Verification items for the finished model (mm, model axes). A direction names the side the tool comes from. Give positions to 0.01 mm unless a question says otherwise; leave off trailing zeros. Loops run counter-clockwise (first coordinate to the right, second up) from the corner with the lowest first, then second, coordinate; pieces in that order, holes last. Notation, with made-up numbers: (3, -11) - (54, -11) arc R27 ccw to (54, 21) - close; hole circle Ø9 at (64, 4). An arc over 180 degrees is marked (long way). Answer in a Markdown table with one row per item.
```python
from build123d import *

# Parameters (mm, degrees)
RESSALTO_EXTRUS_O1_DEPTH = 10
ESBO_O2_R                = 2.2
CORTE_EXTRUS_O1_DEPTH    = 10


with BuildPart() as part:
    # Esboço1 → Ressalto-extrusão1 (new body)
    with BuildSketch(Plane.XY):
        with BuildLine():
            Line((-36, 19), (-19, 19))
            Line((-19, 19), (-19, 0))
            ThreePointArc((-19, 0), (0, -19), (19, 0))
            Line((19, 0), (19, 19))
            Line((19, 19), (36, 19))
            Line((36, 19), (36, 12))
            Line((36, 12), (24, 12))
            Line((24, 12), (24, 0))
            ThreePointArc((24, 0), (0, -24), (-24, 0))
            Line((-24, 0), (-24, 12))
            Line((-24, 12), (-36, 12))
            Line((-36, 12), (-36, 19))
        make_face()
    extrude(amount=RESSALTO_EXTRUS_O1_DEPTH)

    # Esboço2 → Corte-extrusão1 (cut)
    with BuildSketch(Plane(origin=(0, 19, 0), x_dir=(1, 0, 0), z_dir=(0, 1, 0))):
        with Locations((-30, -5)):
            Circle(ESBO_O2_R)
        with Locations((30, -5)):
            Circle(ESBO_O2_R)
    extrude(amount=-CORTE_EXTRUS_O1_DEPTH, mode=Mode.SUBTRACT)


solid = part.part
```
Q1. Sectioned sample at D-D (x = 0). Record the cut outline in (y, z).
Completed:
| item | result |
|---|---|
| outline | (-24, 0) - (-19, 0) - (-19, 10) - (-24, 10) - close |
Q2. Sectioned sample at C-C (y = 9). Record the cut outline in (x, z), and give its area (3 significant figures).
Completed:
| item | result |
|---|---|
| outline | (-24, 0) - (-19, 0) - (-19, 10) - (-24, 10) - close; (19, 0) - (24, 0) - (24, 10) - (19, 10) - close |
| area | 100 mm^2 |
Q3. Go/stop test with flat-tipped pins: P1, Ø6, axis at x = -16, z = 6, coming from the -Y side; P2, Ø1.5, axis at x = 8, z = 3, coming from the -Y side; P3, Ø5.5, axis at x = -30, z = 5, coming from the -Y side; P4, Ø8, axis at x = -6.5, y = -13, coming from the +Z side. Record where each tip stops, or that it passes through.
Completed:
| item | result |
|---|---|
| P1 | y = -20.17 |
| P2 | y = -22.88 |
| P3 | y = 12 |
| P4 | through |
Q4. Thickness scan on line 1 (Z direction, x = -30, y = 17); line 2 (X direction, y = 17.25, z = 5); line 3 (X direction, y = 10, z = 1.5). Record the ranges inside material, lowest first.
Completed:
| item | result |
|---|---|
| line 1 | 0 to 2.8, 7.2 to 10 |
| line 2 | -36 to -32.2, -27.8 to -19, 19 to 27.8, 32.2 to 36 |
| line 3 | -24 to -19, 19 to 24 |
Q5. Sectioned sample at B-B (z = 5). Record the cut outline in (x, y), and give its area (3 significant figures).
Completed:
| item | result |
|---|---|
| outline | (-36, 12) - (-32.2, 12) - (-32.2, 19) - (-36, 19) - close; (-27.8, 12) - (-24, 12) - (-24, 0) arc R24 ccw to (24, 0) - (24, 12) - (27.8, 12) - (27.8, 19) - (19, 19) - (19, 0) arc R19 cw to (-19, 0) - (-19, 19) - (-27.8, 19) - close; (32.2, 12) - (36, 12) - (36, 19) - (32.2, 19) - close |
| area | 634 mm^2 |
Q6. Tool access check on faces 4 (the face through (-24, 6, 5)), 5 (the face through (31.4, 12, 2.7)), 6 (the face through (-19, 10, 5)). Record the directions out of +Z, -Z, +X, -X, +Y, -Y that give a thin tool (end or side, any length) a straight path to the whole face; none if there is none.
Completed:
| item | result |
|---|---|
| face 4 | +Z, -Z, -X, -Y |
| face 5 | +Z, -Z, +X, -Y |
| face 6 | +Z, -Z, +Y |
Q7. Draft check along X on faces 1 (the face through (19, 9, 5)), 2 (the face through (27, 19, 5)), 3 (the face through (36, 16, 5)). Enter one of: +X half, -X half, draft (parallel to the pull), parting line (faces both ways), or undercut.
Completed:
| item | result |
|---|---|
| face 1 | undercut |
| face 2 | draft |
| face 3 | +X half |
Q8. Sectioned sample at A-A (x = 30). Record the cut outline in (y, z), and give its area (3 significant figures).
Completed:
| item | result |
|---|---|
| outline | (12, 0) - (19, 0) - (19, 2.8) - (12, 2.8) - close; (12, 7.2) - (19, 7.2) - (19, 10) - (12, 10) - close |
| area | 39.2 mm^2 |
